Read the model definition and answer for the solid it produces. Units are mm, in the model's axes. Face numbers are marked on the shaded views. Coordinates: 2 decimals unless noted, no trailing zeros. Loops run counter-clockwise (first coordinate to the right, second up) from the corner with the lowest first, then second, coordinate; pieces in that order, holes last.
from build123d import *

# Parameters (mm, degrees)
BOSS_EXTRUDE1_DEPTH  = 10
SKETCH2_R            = 15
MOTOR_HOLE_DEPTH     = 11
SCREW_HOLE_DEPTH     = 5
CUT_EXTRUDE3_DEPTH   = 6
LPATTERN1_COUNT      = 2
LPATTERN1_PITCH      = 31
LPATTERN1_COUNT_DIR2 = 2
LPATTERN1_PITCH_DIR2 = 31
CUT_EXTRUDE4_DEPTH   = 6
CUT_EXTRUDE5_DEPTH   = 5
SKETCH8_R            = 2.065
CUT_EXTRUDE6_DEPTH   = 11


with BuildPart() as part:
    # Sketch1 → Boss-Extrude1 (new body)
    with BuildSketch(Plane.XY):
        Polygon((-33.5, 0), (33.5, 0), (33.5, 117.5), (-28.5, 117.5), (-33.5, 112.5), align=None)
    extrude(amount=BOSS_EXTRUDE1_DEPTH)

    # Sketch2 → Motor Hole (cut, through all)
    with BuildSketch(Plane.XY.offset(10)):
        with Locations((0, 44.5)):
            Circle(SKETCH2_R)
    extrude(amount=-MOTOR_HOLE_DEPTH, mode=Mode.SUBTRACT)

    # Sketch3 → Screw Hole (cut)
    with BuildSketch(Plane.XY.offset(10)):
        with BuildLine():
            Line((-12.5, 66), (-12.5, 56))
            ThreePointArc((-12.5, 56), (-15.5, 53), (-18.5, 56))
            Line((-18.5, 56), (-18.5, 66))
            ThreePointArc((-18.5, 66), (-15.5, 69), (-12.5, 66))
        make_face()
    screw_hole = extrude(amount=-SCREW_HOLE_DEPTH, mode=Mode.SUBTRACT)

    # Sketch5 → Cut-Extrude3 (cut, through all)
    with BuildSketch(Plane.XY.offset(5)):
        with BuildLine():
            Line((-17.25, 66), (-17.25, 56))
            ThreePointArc((-17.25, 56), (-15.5, 54.25), (-13.75, 56))
            Line((-13.75, 56), (-13.75, 66))
            ThreePointArc((-13.75, 66), (-15.5, 67.75), (-17.25, 66))
        make_face()
    cut_extrude3 = extrude(amount=-CUT_EXTRUDE3_DEPTH, mode=Mode.SUBTRACT)

    # LPattern1: Screw Hole, Cut-Extrude3 2 × 2
    with Locations(*[(i * LPATTERN1_PITCH, -j * LPATTERN1_PITCH_DIR2, 0) for i in range(LPATTERN1_COUNT) for j in range(LPATTERN1_COUNT_DIR2) if (i, j) != (0, 0)]):
        add(screw_hole, mode=Mode.SUBTRACT)
        add(cut_extrude3, mode=Mode.SUBTRACT)

    # Sketch6 → Cut-Extrude4 (cut)
    with BuildSketch(Plane.XY.offset(10)):
        with BuildLine():
            Line((-20.4, 57.5), (-20.4, 42.5))
            ThreePointArc((-20.4, 42.5), (-25.5, 37.4), (-30.6, 42.5))
            Line((-30.6, 42.5), (-30.6, 57.5))
            ThreePointArc((-30.6, 57.5), (-25.5, 62.6), (-20.4, 57.5))
        make_face()
    cut_extrude4 = extrude(amount=-CUT_EXTRUDE4_DEPTH, mode=Mode.SUBTRACT)

    # Sketch7 → Cut-Extrude5 (cut, through all)
    with BuildSketch(Plane.XY.offset(4)):
        with BuildLine():
            Line((-28.25, 57.5), (-28.25, 42.5))
            ThreePointArc((-28.25, 42.5), (-25.5, 39.75), (-22.75, 42.5))
            Line((-22.75, 42.5), (-22.75, 57.5))
            ThreePointArc((-22.75, 57.5), (-25.5, 60.25), (-28.25, 57.5))
        make_face()
    cut_extrude5 = extrude(amount=-CUT_EXTRUDE5_DEPTH, mode=Mode.SUBTRACT)

    # Mirror1: Cut-Extrude4, Cut-Extrude5 across plane
    add(cut_extrude4.mirror(Plane(origin=(0, 0, 0), x_dir=(0, 0, 1), z_dir=(1, 0, 0))), mode=Mode.SUBTRACT)
    add(cut_extrude5.mirror(Plane(origin=(0, 0, 0), x_dir=(0, 0, 1), z_dir=(1, 0, 0))), mode=Mode.SUBTRACT)

    # Sketch8 → Cut-Extrude6 (cut, through all)
    with BuildSketch(Plane.XY.offset(10)):
        with Locations((23.5, 94)):
            Circle(SKETCH8_R)
        with Locations((23.5, 80)):
            Circle(SKETCH8_R)
    extrude(amount=-CUT_EXTRUDE6_DEPTH, mode=Mode.SUBTRACT)


solid = part.part
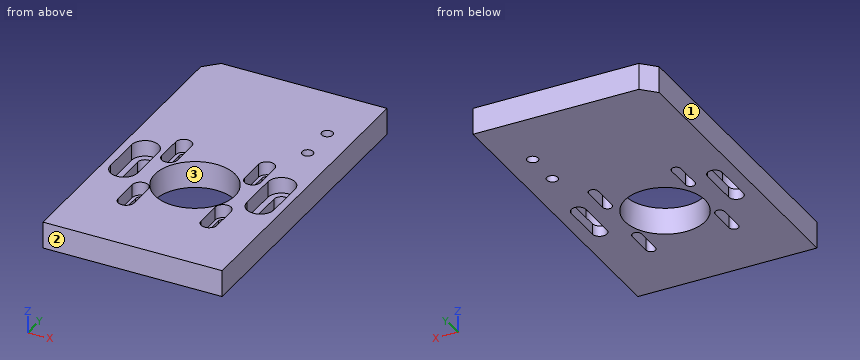
Q1. A cutting plane is placed at B-B (y = 44.5). Give the vertices of the cut face in (x, z).
Findings below:
outline: (-33.5, 0) - (-28.25, 0) - (-28.25, 4) - (-30.6, 4) - (-30.6, 10) - (-33.5, 10) - close; (-22.75, 0) - (-15, 0) - (-15, 10) - (-20.4, 10) - (-20.4, 4) - (-22.75, 4) - close; (15, 0) - (22.75, 0) - (22.75, 4) - (20.4, 4) - (20.4, 10) - (15, 10) - close; (28.25, 0) - (33.5, 0) - (33.5, 10) - (30.6, 10) - (30.6, 4) - (28.25, 4) - close
Q2. Determine the mould class of the marked faces 1, 2 and 3 for opening direction Y: +Y half, -Y half, draft (parallel to the pull), parting line (faces both ways), or undercut.
Findings below:
face 1: draft
face 2: -Y half
face 3: undercut
Q3. A cutting plane is placed at C-C (y = 80). Give the vertices of the cut face in (x, z) (3 decimals).
Findings below:
outline: (-33.5, 0) - (21.435, 0) - (21.435, 10) - (-33.5, 10) - close; (25.565, 0) - (33.5, 0) - (33.5, 10) - (25.565, 10) - close
Q4. Straight lines are drawn through the part: probe 1 along Y at (x, z) = (-15.5, 4.25); probe 2 along Y at (x, z) = (25, 3.5); probe 3 along X at (y, z) = (61, 4.5). For each, find the intervals that lie inside material, in ascending order.
Findings below:
probe 1: y = 0 to 23.25, 36.75 to 54.25, 67.75 to 117.5
probe 2: y = 0 to 39.8, 60.2 to 78.58, 81.42 to 92.58, 95.42 to 117.5
probe 3: x = -33.5 to -29.21, -21.79 to -17.25, -13.75 to 13.75, 17.25 to 21.79, 29.21 to 33.5
Q5. A cutting plane is placed at A-A (x = -25.5). Give the vertices of the cut face in (y, z).
Findings below:
outline: (0, 0) - (39.75, 0) - (39.75, 4) - (37.4, 4) - (37.4, 10) - (0, 10) - close; (60.25, 0) - (117.5, 0) - (117.5, 10) - (62.6, 10) - (62.6, 4) - (60.25, 4) - close
Q6. Flat-ended cylindrical pins translate along their axes: pin 1 Ø2.5 at (x, y) = (23.5, 80) entering from +Z (3 decimals); pin 2 Ø8 at (x, y) = (25.5, 51) entering from +Z; pin 3 Ø3 at (x, y) = (15, 61.5) entering from +Z. Find the tip coordinate at first contact, or state that the pin passes through.
Findings below:
pin 1: passes through
pin 2: stops at z = 4
pin 3: stops at z = 5
